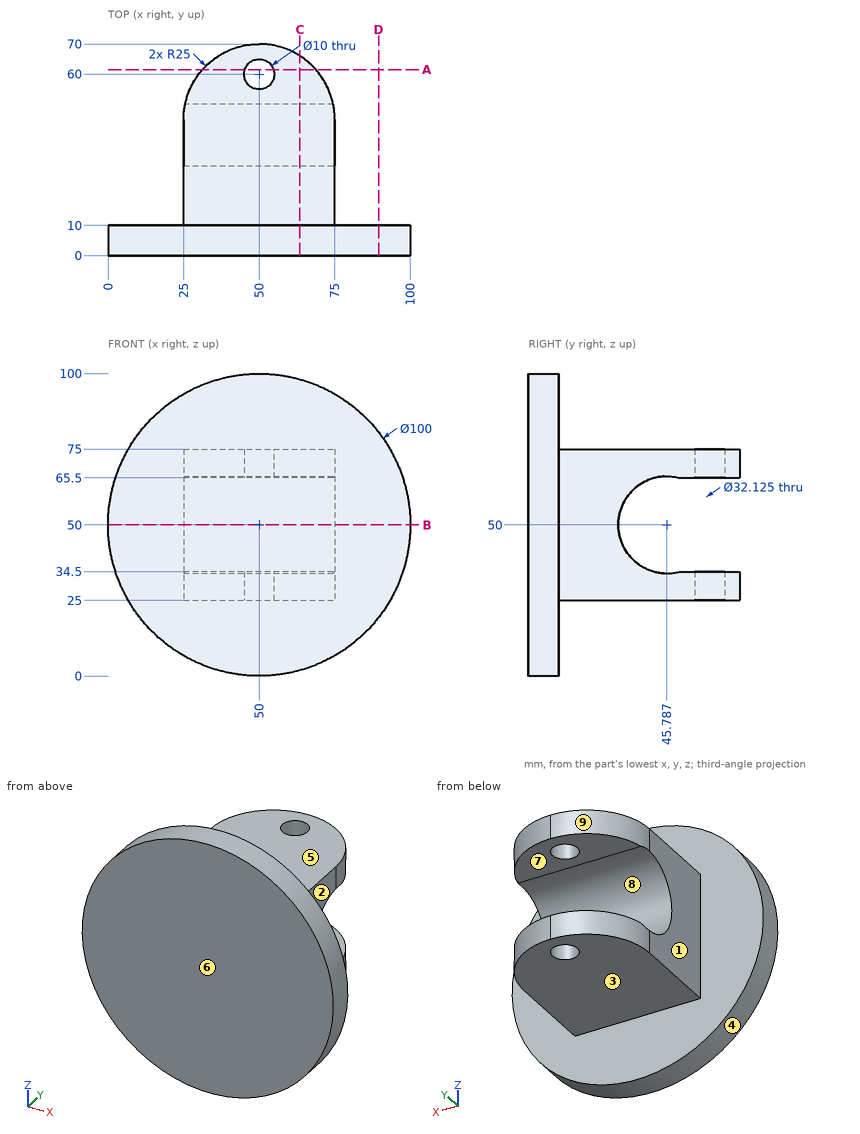
Geometry check sheet. Reference: drawing and pictorial views, mm from the part's lowest x, y, z. A direction names the side the tool comes from. Round coordinates to 2 decimals unless told otherwise and drop trailing zeros. Loops run counter-clockwise (first coordinate to the right, second up) from the corner with the lowest first, then second, coordinate; pieces in that order, holes last. Notation, with made-up numbers: M -16.75,9.25 L 25.25,9.25 A21 ccw 25.25,19.25 Z; hole C 87,-9.5 d5. An arc over 180 degrees is marked long. One line per item, written item: value.
(1) Sectioned sample at B-B, the plane z = 50. Record the cut outline in (x, y) (1 decimal), then the cut area to 3 significant figures.
Computed values:
outline: M 0,0 L 100,0 L 100,10 L 75,10 L 75,29.7 L 25,29.7 L 25,10 L 0,10 Z
area: 1,990 mm^2
(2) Sectioned sample at A-A, the plane y = 61.5. Record the cut outline in (x, z).
Computed values:
outline: M 31.22,25 L 45.23,25 L 45.23,34.5 L 31.22,34.5 Z; M 31.22,65.5 L 45.23,65.5 L 45.23,75 L 31.22,75 Z; M 54.77,25 L 68.78,25 L 68.78,34.5 L 54.77,34.5 Z; M 54.77,65.5 L 68.78,65.5 L 68.78,75 L 54.77,75 Z
(3) Access from +Z, -Z, +X, -X, +Y, -Y to the whole of each face (thin tool, end or side, straight path). Record for the marked faces 1, 2, 3, 4 and 5.
Computed values:
face 1: +Z, -Z, -X, +Y
face 2: +Z, -Z, +X, +Y
face 3: -Z, +X, -X, +Y
face 4: +Y, -Y
face 5: +Z, +X, -X, +Y
(4) Thickness scan on line 1 (Z direction, x = 61.5, y = 45); line 2 (Y direction, x = 50, z = 31.5); line 3 (Y direction, x = 22.5, z = 86). Record the ranges inside material, lowest first.
Computed values:
line 1: z = 25 to 33.96, 66.04 to 75
line 2: y = 0 to 55, 65 to 70
line 3: y = 0 to 10
(5) Depth check by flat-ended pin: pin 1 Ø25 at (x, y) = (57, 54) entering from +Z; pin 2 Ø4 at (y, z) = (35, 62) entering from -X; pin 3 Ø3 at (x, z) = (36, 23) entering from +Y; pin 4 Ø8 at (x, y) = (50, 60) entering from +Z (3 decimals). Enter the tip coordinate at first touch or a pass-through.
Computed values:
pin 1: stops at z = 75
pin 2: stops at x = 25
pin 3: stops at y = 10
pin 4: passes through
(6) Sectioned sample at C-C, the plane x = 63.5. Record the cut outline in (y, z) (1 decimal).
Computed values:
outline: M 0,1.9 L 10,1.9 L 10,25 L 66,25 L 66,34.5 L 50,34.5 A16.1 cw long 50,65.5 L 66,65.5 L 66,75 L 10,75 L 10,98.1 L 0,98.1 Z
(7) Sectioned sample at D-D, the plane x = 89.5. Record the cut outline in (y, z) (1 decimal).
Computed values:
outline: M 0,19.3 L 10,19.3 L 10,80.7 L 0,80.7 Z
(8) Release check for a two-part mould opening along Y. For the marked faces 6, 7, 8 and 9 record: +Y half, -Y half, draft (parallel to the pull), parting line (faces both ways), or undercut.
Computed values:
face 6: -Y half
face 7: draft
face 8: undercut
face 9: +Y half
